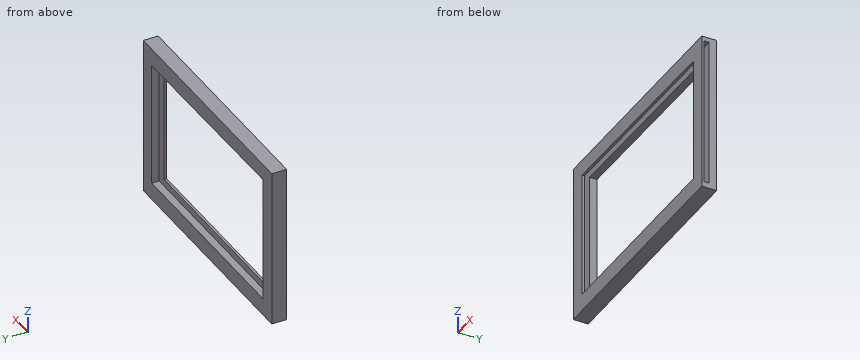
from build123d import *

# Parameters (mm, degrees)
F0_W     = 127
F0_H     = 76.2
F1_DEPTH = 2.54
F2_W     = 121.95362
F2_H     = 81.28
F3_DEPTH = 3.81
F5_DEPTH = 25.4


with BuildPart() as f1:
    # F0 (on Front) → F1 (new body)
    with BuildSketch(Plane.XZ):
        Rectangle(F0_W, F0_H)
    extrude(amount=F1_DEPTH)


with BuildPart() as f3:
    # F2 (on Front) → F3 (new body, symmetric)
    with BuildSketch(Plane.XZ):
        with Locations((-4.591286, -0.313837)):
            Rectangle(F2_W, F2_H)
    extrude(amount=F3_DEPTH, both=True)


with BuildPart() as f5_tool:
    # F4 (on face) → F5 (new body)
    with BuildSketch(Plane.XZ.offset(3.81)):
        Polygon((48.386987, 31.428229), (-57.210241, 32.319993), (-57.210241, -32.189324), (48.386987, -32.189324), align=None)
    extrude(amount=-F5_DEPTH)


with BuildPart() as f1_1:
    add(f1.part)

    # F5: cut by f5_tool
    add(f5_tool.part, mode=Mode.SUBTRACT)


with BuildPart() as f3_1:
    add(f3.part)

    # F5: cut by f5_tool
    add(f5_tool.part, mode=Mode.SUBTRACT)

    # F6: cut F1
    add(f1_1.part, mode=Mode.SUBTRACT)


solid = f3_1.part
Geometry: final body of the model. Coordinates: model frame, mm. Give positions to 0.01 mm unless a question says otherwise; leave off trailing zeros. Write each loop counter-clockwise with the first axis right and the second up, starting at its lowest first coordinate (ties: lowest second). Pieces come first, ordered by that corner, then holes.
(1) Cut plane C-C, the plane y = 2. Return loops of the section in (x, z).
(2) Cut plane A-A, the plane z = 7.5. Return loops of the section in (x, y).
(3) Ray query, line 1 (Z direction, x = 19.5, y = -1); line 2 (Z direction, x = -54, y = -3); line 3 (X direction, y = 3.25, z = 26). Return the intervals inside material, ascending.
(4) Cut plane D-D, the plane x = -37. Return loops of the section in (y, z).
(5) Cut plane B-B, the plane x = 42.5. Return loops of the section in (y, z), then the cut area to 3 significant figures.
Values follow:
1. outline: (-65.57, -40.95) - (56.39, -40.95) - (56.39, 40.33) - (-65.57, 40.33) - close; hole (-57.21, -32.19) - (48.39, -32.19) - (48.39, 31.43) - (-57.21, 32.32) - close
2. outline: (-65.57, -3.81) - (-57.21, -3.81) - (-57.21, -2.54) - (-63.5, -2.54) - (-63.5, 0) - (-57.21, 0) - (-57.21, 3.81) - (-65.57, 3.81) - close; (48.39, -3.81) - (56.39, -3.81) - (56.39, -2.54) - (48.39, -2.54) - close; (48.39, 0) - (56.39, 0) - (56.39, 3.81) - (48.39, 3.81) - close
3. line 1: z = -40.95 to -38.1, 38.1 to 40.33
3. line 2: z = -40.95 to -32.19, 32.29 to 40.33
3. line 3: x = -65.57 to -57.21, 48.39 to 56.39
4. outline: (-3.81, -40.95) - (3.81, -40.95) - (3.81, -32.19) - (0, -32.19) - (0, -38.1) - (-2.54, -38.1) - (-2.54, -32.19) - (-3.81, -32.19) - close; (-3.81, 32.15) - (-2.54, 32.15) - (-2.54, 38.1) - (0, 38.1) - (0, 32.15) - (3.81, 32.15) - (3.81, 40.33) - (-3.81, 40.33) - close
5. outline: (-3.81, -40.95) - (3.81, -40.95) - (3.81, -32.19) - (0, -32.19) - (0, -38.1) - (-2.54, -38.1) - (-2.54, -32.19) - (-3.81, -32.19) - close; (-3.81, 31.48) - (-2.54, 31.48) - (-2.54, 38.1) - (0, 38.1) - (0, 31.48) - (3.81, 31.48) - (3.81, 40.33) - (-3.81, 40.33) - close
5. area: 102 mm2
